from build123d import *

# Parameters (mm, degrees)
SKETCH_1_W               = 78
SKETCH_1_H               = 101
EXTRUDE_1_DEPTH          = 121
SKETCH_4_W               = 86
SKETCH_4_H               = 86
EXTRUDE_2_DEPTH          = 127
CUT_EXTRUDE_1_DEPTH      = 189.857088826
CUT_EXTRUDE_1_DEPTH_BACK = 189.857088826
SKETCH_5_R               = 7
CHAMFER_1_SIZE           = 5
CUT_EXTRUDE_2_REACH      = 269.436
SKETCH_6_R               = 3
SKETCH_7_R               = 3
CUT_EXTRUDE_3_DEPTH      = 181.607308822
SKETCH_8_R               = 46.5
SKETCH_8_R_2             = 36.5
CUT_EXTRUDE_1_2_DEPTH    = 3
CUT_EXTRUDE_START        = -3
SKETCH_9_R               = 46.5
SKETCH_9_R_2             = 36.5
CUT_EXTRUDE_2_2_DEPTH    = 3
KEYWAY_DEPTH             = 214.350603768


with BuildPart() as part:
    # 草图1 → 凸台-拉伸1 (new body)
    with BuildSketch(Plane(origin=(0, 0, 0), x_dir=(1, 0, 0), z_dir=(0, 1, 0))):
        with Locations((0, 50.5)):
            Rectangle(SKETCH_1_W, SKETCH_1_H)
    extrude(amount=EXTRUDE_1_DEPTH)

    # 草图4 → 凸台-拉伸2 (add)
    with BuildSketch(Plane.XY):
        with Locations((0, 90)):
            Rectangle(SKETCH_4_W, SKETCH_4_H)
    extrude(amount=EXTRUDE_2_DEPTH)

    # 草图5 → Cut-Extrude 1 (cut, two sides: drawn at the far end of the back side and taken through both)
    with BuildSketch(Plane(origin=(0, 0, 0), x_dir=(0, 0, -1), z_dir=(1, 0, 0)).offset(-CUT_EXTRUDE_1_DEPTH_BACK)):
        with Locations(Location((50.5, 50, 0), (0, 0, 180))):
            Circle(SKETCH_5_R)
    extrude(amount=CUT_EXTRUDE_1_DEPTH + CUT_EXTRUDE_1_DEPTH_BACK, mode=Mode.SUBTRACT)

    # 倒角1
    # the kernel refuses this chamfer: 5 mm, written as the material it takes off along each edge
    with BuildSketch(Plane(origin=(39.666666667, 50.333333333, 123.666666667), x_dir=(0.7071067811865475, -2.009718347115232e-15, -0.7071067811865475), z_dir=(0.5773502691896247, -0.5773502691896264, 0.5773502691896264)), Plane(origin=(39.666666667, 129.666666667, 123.666666667), x_dir=(-0.7071067811865475, 2.009718347115232e-15, 0.7071067811865475), z_dir=(0.5773502691896272, 0.5773502691896246, 0.5773502691896255))) as chamfer_1_piece_1:
        Polygon((-3.535533906, 2.041241452), (3.535533906, 2.041241452), (0, -4.082482905), align=None)
    extrude(amount=6.350852961, mode=Mode.SUBTRACT)
    with BuildSketch(Plane(origin=(-39.666666667, 129.666666667, 123.666666667), x_dir=(0.7071067811865475, 0, 0.7071067811865475), z_dir=(-0.5773502691896257, 0.5773502691896257, 0.5773502691896257)), Plane(origin=(-39.666666667, 50.333333333, 123.666666667), x_dir=(-0.7071067811865475, 0, -0.7071067811865475), z_dir=(-0.5773502691896261, -0.5773502691896253, 0.5773502691896261))) as chamfer_1_piece_2:
        Polygon((-3.535533906, -2.041241452), (3.535533906, -2.041241452), (0, 4.082482905), align=None)
    extrude(amount=6.350852961, mode=Mode.SUBTRACT)
    with BuildSketch(Plane(origin=(43, 47, 0), x_dir=(-0.9996219169112968, -0.027495876610586317, 0), z_dir=(0, 0, 1))) as chamfer_1_piece_3:
        Polygon((CHAMFER_1_SIZE * 0.999621916911, -CHAMFER_1_SIZE * 0.0274958766106), (-CHAMFER_1_SIZE * 0.0274958766106, -CHAMFER_1_SIZE * 0.999621916911), (0, 0), align=None)
    extrude(amount=139.85841494, mode=Mode.SUBTRACT)
    with BuildSketch(Plane(origin=(43, 133, -12.85841494), x_dir=(0.027495876610586206, -0.9996219169112968, 0), z_dir=(0, 0, 1))) as chamfer_1_piece_4:
        Polygon((CHAMFER_1_SIZE * 0.999621916911, -CHAMFER_1_SIZE * 0.0274958766106), (-CHAMFER_1_SIZE * 0.0274958766106, -CHAMFER_1_SIZE * 0.999621916911), (0, 0), align=None)
    extrude(amount=152.71682988, mode=Mode.SUBTRACT)
    with BuildSketch(Plane(origin=(-43, 133, -12.85841494), x_dir=(-0.027495876610586355, -0.9996219169112968, 0), z_dir=(0, 0, 1))) as chamfer_1_piece_5:
        Polygon((CHAMFER_1_SIZE * 0.999621916911, CHAMFER_1_SIZE * 0.0274958766106), (-CHAMFER_1_SIZE * 0.0274958766106, CHAMFER_1_SIZE * 0.999621916911), (0, 0), align=None)
    extrude(amount=152.71682988, mode=Mode.SUBTRACT)
    with BuildSketch(Plane(origin=(-43, 47, 0), x_dir=(0.9996219169112968, -0.027495876610586355, 0), z_dir=(0, 0, 1))) as chamfer_1_piece_6:
        Polygon((CHAMFER_1_SIZE * 0.999621916911, CHAMFER_1_SIZE * 0.0274958766106), (-CHAMFER_1_SIZE * 0.0274958766106, CHAMFER_1_SIZE * 0.999621916911), (0, 0), align=None)
    extrude(amount=139.85841494, mode=Mode.SUBTRACT)
    with BuildSketch(Plane(origin=(43, 145.85841494, 127), x_dir=(0.027495876610586282, 0, -0.9996219169112968), z_dir=(0, -1, 0)), Plane(origin=(-43, 34.14158506, 127), x_dir=(-0.027495876610586282, 0, -0.9996219169112968), z_dir=(0, 1, 0)), Plane(origin=(55.85841494, 47, 127), x_dir=(0, -0.027495876610586282, -0.9996219169112968), z_dir=(-1, 0, 0))) as chamfer_1_piece_7:
        Polygon((CHAMFER_1_SIZE * 0.999621916911, -CHAMFER_1_SIZE * 0.0274958766106), (-CHAMFER_1_SIZE * 0.0274958766106, -CHAMFER_1_SIZE * 0.999621916911), (0, 0), align=None)
    extrude(amount=111.71682988, mode=Mode.SUBTRACT)
    with BuildSketch(Plane(origin=(-55.85841494, 133, 127), x_dir=(0, -0.9996219169112968, 0.027495876610587663), z_dir=(1, 0, 0))) as chamfer_1_piece_8:
        Polygon((CHAMFER_1_SIZE * 0.999621916911, CHAMFER_1_SIZE * 0.0274958766106), (-CHAMFER_1_SIZE * 0.0274958766106, CHAMFER_1_SIZE * 0.999621916911), (0, 0), align=None)
    extrude(amount=111.71682988, mode=Mode.SUBTRACT)

    # 草图6 → Cut-Extrude 2 (cut, up to next)
    with BuildSketch(Plane(origin=(0, 0, -101), x_dir=(-1, 0, 0), z_dir=(0, 0, -1)), mode=Mode.PRIVATE) as cut_extrude_2_sk1:
        with Locations((-30, 15)):
            Circle(SKETCH_6_R)
    cut_extrude_2_tool1 = extrude(cut_extrude_2_sk1.sketch, amount=-CUT_EXTRUDE_2_REACH, mode=Mode.PRIVATE) & part.part
    # 草图6 → Cut-Extrude 2 (cut, up to next)
    with BuildSketch(Plane(origin=(0, 0, -101), x_dir=(-1, 0, 0), z_dir=(0, 0, -1)), mode=Mode.PRIVATE) as cut_extrude_2_sk2:
        with Locations((30, 15)):
            Circle(SKETCH_6_R)
    cut_extrude_2_tool2 = extrude(cut_extrude_2_sk2.sketch, amount=-CUT_EXTRUDE_2_REACH, mode=Mode.PRIVATE) & part.part
    # 草图6 → Cut-Extrude 2 (cut, up to next)
    with BuildSketch(Plane(origin=(0, 0, -101), x_dir=(-1, 0, 0), z_dir=(0, 0, -1)), mode=Mode.PRIVATE) as cut_extrude_2_sk3:
        with Locations((-30, 105)):
            Circle(SKETCH_6_R)
    cut_extrude_2_tool3 = extrude(cut_extrude_2_sk3.sketch, amount=-CUT_EXTRUDE_2_REACH, mode=Mode.PRIVATE) & part.part
    # 草图6 → Cut-Extrude 2 (cut, up to next)
    with BuildSketch(Plane(origin=(0, 0, -101), x_dir=(-1, 0, 0), z_dir=(0, 0, -1)), mode=Mode.PRIVATE) as cut_extrude_2_sk4:
        with Locations((30, 105)):
            Circle(SKETCH_6_R)
    cut_extrude_2_tool4 = extrude(cut_extrude_2_sk4.sketch, amount=-CUT_EXTRUDE_2_REACH, mode=Mode.PRIVATE) & part.part
    add(cut_extrude_2_tool1.solids().sort_by_distance((30, 15, -101))[0], mode=Mode.SUBTRACT)
    add(cut_extrude_2_tool2.solids().sort_by_distance((-30, 15, -101))[0], mode=Mode.SUBTRACT)
    add(cut_extrude_2_tool3.solids().sort_by_distance((30, 105, -101))[0], mode=Mode.SUBTRACT)
    add(cut_extrude_2_tool4.solids().sort_by_distance((-30, 105, -101))[0], mode=Mode.SUBTRACT)

    # 草图7 → 切除-拉伸3 (cut, through all)
    with BuildSketch(Plane(origin=(0, 121, 0), x_dir=(1, 0, 0), z_dir=(0, 1, 0))):
        with Locations((30, 85.5)):
            Circle(SKETCH_7_R)
        with Locations((30, 15.5)):
            Circle(SKETCH_7_R)
        with Locations((-30, 15.5)):
            Circle(SKETCH_7_R)
        with Locations((-30, 85.5)):
            Circle(SKETCH_7_R)
    extrude(amount=-CUT_EXTRUDE_3_DEPTH, mode=Mode.SUBTRACT)

    # 草图8 → Cut-Extrude 1 2 (cut)
    with BuildSketch(Plane.ZY.offset(39)):
        with Locations((-50.5, 50)):
            Circle(SKETCH_8_R)
        with Locations((-50.5, 50)):
            Circle(SKETCH_8_R_2, mode=Mode.SUBTRACT)
    extrude(amount=-CUT_EXTRUDE_1_2_DEPTH, mode=Mode.SUBTRACT)

    # 草图9 → Cut-Extrude 2 2 (cut)
    with BuildSketch(Plane(origin=(39, 0, 0), x_dir=(0, 0, -1), z_dir=(1, 0, 0)).offset(CUT_EXTRUDE_START)):
        with Locations((50.5, 50)):
            Circle(SKETCH_9_R)
        with Locations((50.5, 50)):
            Circle(SKETCH_9_R_2, mode=Mode.SUBTRACT)
    extrude(amount=CUT_EXTRUDE_2_2_DEPTH, mode=Mode.SUBTRACT)

    # KeySketch → Keyway (cut, through all)
    with BuildSketch(Plane(origin=(-39, 56.979737296, -54.70140282), x_dir=(0, 0, 1), z_dir=(-1, 0, 0))):
        with BuildLine():
            Line((0.196955351, 1.08031236), (-0.204032077, 4.370687514))
            Line((-0.204032077, 4.370687514), (5.7519036, 5.096518221))
            Line((5.7519036, 5.096518221), (6.152891028, 1.806143068))
            ThreePointArc((6.152891028, 1.806143068), (5.290148882, -15.913640811), (0.196955351, 1.08031236))
        make_face()
    extrude(amount=-KEYWAY_DEPTH, mode=Mode.SUBTRACT)


solid = part.part
Read the model definition and answer for the solid it produces. Units are mm, in the model's axes. A direction names the side the tool comes from. Round coordinates to 2 decimals unless told otherwise and drop trailing zeros. Order: outer loops, then holes, each group sorted by start corner. A loop starts at its lowest first (then second) coordinate and runs counter-clockwise, first axis right, second up.
1) The part is cut by section A-A on x = -1.5. Write down the section's boundary in (y, z), plus the area to 3 significant figures.
2) The mould has two halves that part along Z. Classify faces 6 (the face through (-40, 130, 123)), 7 (the face through (43, 89, 60)), 8 (the face through (27.6, 60.6, -13.7)), 9 (the face through (-28.39, 113.11, -18.03)): released by +Z, released by -Z, zero draft, split by the parting line, or undercut.
3) Straight lines are drawn through the part: L1, parallel to X at y = 44, z = -15.5; L2, parallel to X at y = 105, z = 48; L3, parallel to Y at x = 30, z = -10. For each, find the intervals that lie inside material, in ascending order.
4) The part is cut by section B-B on x = 30. Give the number of separate pieces and of enclosed holes in the cut face, plus the area to 3 significant figures.
5) For faces 1 (the face through (-1, 121, -51)), 2 (the face through (39, 100, -50)), 3 (the face through (30.65, 102.07, -50.99)), 4 (the face through (-1, 47, 60)), 5 (the face through (-37.521, 32.19, -7.546)), determine the directions among +Z, -Z, +X, -X, +Y, -Y from which every point of the face is accessible in a straight line to the end or side of a thin tool.
6) The part is cut by section D-D on z = 46. Write down the section's boundary in (x, y).
7) Flat-ended cylindrical pins translate along their axes: pin 1 (5.5 mm diameter, centred on x = -30, z = -15.5, fed in from +Y); pin 2 (6 mm diameter, centred on x = 19.5, z = -48, fed in from +Y); pin 3 (9.5 mm diameter, centred on x = -30, y = 105, fed in from +Z). Find the tip coordinate at first contact, or state that the pin passes through.
Resolved:
1. outline: (0, -101) - (121, -101) - (121, 0) - (133, 0) - (133, 122) - (128, 127) - (52, 127) - (47, 122) - (47, 0) - (0, 0) - close; hole (58.06, -54.5) - (61.35, -54.91) - (62.08, -48.95) - (58.79, -48.55) arc R9 ccw (long way) to start
1. area: 22,800 mm2
2. face 6: released by +Z
2. face 7: zero draft
2. face 8: undercut
2. face 9: undercut
3. L1: x = -39 to -33, -27 to 27, 33 to 39
3. L2: x = -43 to -33, -27 to 27, 33 to 43
3. L3: y = 0 to 12, 18 to 102, 108 to 121
4. separate pieces: 9
4. enclosed holes: 1
4. area: 19,600 mm2
5. face 1: -Z, +X, -X, +Y
5. face 2: -Z, +X, +Y, -Y
5. face 3: +Z, -Z
5. face 4: +Z, +X, -X, -Y
5. face 5: -X
6. outline: (-43, 52) - (-38, 47) - (38, 47) - (43, 52) - (43, 128) - (38, 133) - (-38, 133) - (-43, 128) - close; hole circle Ø6 at (-30, 105); hole circle Ø6 at (30, 105)
7. pin 1: passes through
7. pin 2: stops at y = 121
7. pin 3: stops at z = 127
